Input: part model. Units: mm. Frame: model coordinates. Give positions to 0.01 mm unless a question says otherwise; leave off trailing zeros. Loops run counter-clockwise (first coordinate to the right, second up) from the corner with the lowest first, then second, coordinate; pieces in that order, holes last. Notation, with made-up numbers: (67, 68) -> (111, 68) arc R26 ccw to (111, 94) -> close; hole circle Ø1 at (26.5, 44). An arc over 180 degrees is marked (long way). Answer in a Markdown table with one row per item. Add a question column.
```python
from build123d import *

# Parameters (mm, degrees)
SKETCH1_W           = 17.78
SKETCH1_H           = 33.1
BOSS_EXTRUDE1_DEPTH = 0.8
FILLET1_R           = 0.5
SKETCH2_W           = 9
SKETCH2_H           = 7.3
CUT_EXTRUDE1_DEPTH  = 0.8
SKETCH2_3_W         = 9
SKETCH2_3_H         = 7.3
BOSS_EXTRUDE2_DEPTH = 2.4
SKETCH4_W           = 9
SKETCH4_H           = 2.4
BOSS_EXTRUDE3_DEPTH = 1.524
SKETCH5_W           = 9
SKETCH5_H           = 8.824
BOSS_EXTRUDE4_DEPTH = 0.8
SKETCH6_R           = 0.5
CUT_EXTRUDE2_DEPTH  = 1.524
FILLET2_START       = 8
FILLET2_DEPTH       = 11
FILLET2_START_2     = 16.55
FILLET2_2_DEPTH     = 2.45
CUT_EXTRUDE5_START  = -7.3
CUT_EXTRUDE5_DEPTH  = 7.3


with BuildPart() as part:
    # Sketch1 → Boss-Extrude1 (new body)
    with BuildSketch(Plane(origin=(0, 0, 0), x_dir=(1, 0, 0), z_dir=(0, 1, 0))):
        Rectangle(SKETCH1_W, SKETCH1_H)
    extrude(amount=BOSS_EXTRUDE1_DEPTH)

    # Fillet1
    fillet1_edges = [part.edges().sort_by_distance(p)[0] for p in [
        (-8.89, 0.4, -16.55),
        (8.89, 0.4, -16.55),
        (8.89, 0.4, 16.55),
        (-8.89, 0.4, 16.55),
    ]]
    fillet(fillet1_edges, radius=FILLET1_R)

    # Sketch2 → Cut-Extrude1 (cut)
    with BuildSketch(Plane(origin=(0, 0.8, 0), x_dir=(1, 0, 0), z_dir=(0, 1, 0))):
        with Locations((0, -12.9)):
            Rectangle(SKETCH2_W, SKETCH2_H)
    extrude(amount=-CUT_EXTRUDE1_DEPTH, mode=Mode.SUBTRACT)



with BuildPart() as body_2:
    # Sketch2<3> → Boss-Extrude2 (new body)
    with BuildSketch(Plane(origin=(0, 0.8, 0), x_dir=(1, 0, 0), z_dir=(0, 1, 0))):
        with Locations((0, -12.9)):
            Rectangle(SKETCH2_3_W, SKETCH2_3_H)
    extrude(amount=BOSS_EXTRUDE2_DEPTH)

    # Sketch4 → Boss-Extrude3 (add)
    with BuildSketch(Plane.XY.offset(16.55)):
        with Locations((0, 2)):
            Rectangle(SKETCH4_W, SKETCH4_H)
    extrude(amount=BOSS_EXTRUDE3_DEPTH)


with BuildPart() as part_1:
    add(part.part)

    add(body_2.part)  # Boss-Extrude4 merges body 2
    # Sketch5 → Boss-Extrude4 (add)
    with BuildSketch(Plane.XZ.offset(-0.8)):
        with Locations((0, 13.662)):
            Rectangle(SKETCH5_W, SKETCH5_H)
    extrude(amount=BOSS_EXTRUDE4_DEPTH)

    # Sketch6 → Cut-Extrude2 (cut)
    with BuildSketch(Plane(origin=(0, 0.8, 0), x_dir=(1, 0, 0), z_dir=(0, 1, 0))):
        with Locations(Location((-7.62, 15.28, 0), (0, 0, 270))):
            Circle(SKETCH6_R)
        with Locations(Location((7.62, 15.28, 0), (0, 0, 270))):
            Circle(SKETCH6_R)
        with Locations(Location((7.62, 12.74, 0), (0, 0, 270))):
            Circle(SKETCH6_R)
        with Locations(Location((7.62, 10.2, 0), (0, 0, 270))):
            Circle(SKETCH6_R)
        with Locations(Location((7.62, 7.66, 0), (0, 0, 270))):
            Circle(SKETCH6_R)
        with Locations(Location((7.62, 5.12, 0), (0, 0, 270))):
            Circle(SKETCH6_R)
        with Locations(Location((7.62, 2.58, 0), (0, 0, 270))):
            Circle(SKETCH6_R)
        with Locations(Location((7.62, 0.04, 0), (0, 0, 270))):
            Circle(SKETCH6_R)
        with Locations(Location((7.62, -2.5, 0), (0, 0, 270))):
            Circle(SKETCH6_R)
        with Locations(Location((7.62, -5.04, 0), (0, 0, 270))):
            Circle(SKETCH6_R)
        with Locations(Location((7.62, -7.58, 0), (0, 0, 270))):
            Circle(SKETCH6_R)
        with Locations(Location((7.62, -10.12, 0), (0, 0, 270))):
            Circle(SKETCH6_R)
        with Locations(Location((7.62, -12.66, 0), (0, 0, 270))):
            Circle(SKETCH6_R)
        with Locations(Location((7.62, -15.2, 0), (0, 0, 270))):
            Circle(SKETCH6_R)
        with Locations(Location((-7.62, 12.74, 0), (0, 0, 270))):
            Circle(SKETCH6_R)
        with Locations(Location((-7.62, 10.2, 0), (0, 0, 270))):
            Circle(SKETCH6_R)
        with Locations(Location((-7.62, 7.66, 0), (0, 0, 270))):
            Circle(SKETCH6_R)
        with Locations(Location((-7.62, 5.12, 0), (0, 0, 270))):
            Circle(SKETCH6_R)
        with Locations(Location((-7.62, 2.58, 0), (0, 0, 270))):
            Circle(SKETCH6_R)
        with Locations(Location((-7.62, 0.04, 0), (0, 0, 270))):
            Circle(SKETCH6_R)
        with Locations(Location((-7.62, -2.5, 0), (0, 0, 270))):
            Circle(SKETCH6_R)
        with Locations(Location((-7.62, -5.04, 0), (0, 0, 270))):
            Circle(SKETCH6_R)
        with Locations(Location((-7.62, -7.58, 0), (0, 0, 270))):
            Circle(SKETCH6_R)
        with Locations(Location((-7.62, -10.12, 0), (0, 0, 270))):
            Circle(SKETCH6_R)
        with Locations(Location((-7.62, -12.66, 0), (0, 0, 270))):
            Circle(SKETCH6_R)
        with Locations(Location((-7.62, -15.2, 0), (0, 0, 270))):
            Circle(SKETCH6_R)
    extrude(amount=-CUT_EXTRUDE2_DEPTH, mode=Mode.SUBTRACT)

    # Fillet2: read off the stored shape, not the designer's step
    # Fillet2 outline → Fillet2 (cut)
    with BuildSketch(Plane.XY.offset(FILLET2_START)):
        with BuildLine():
            ThreePointArc((-4.5, 2.2), (-4.207106781, 2.907106781), (-3.5, 3.2))
            Line((-3.5, 3.2), (-4.5, 3.2))
            Line((-4.5, 3.2), (-4.5, 2.2))
        make_face()
        with BuildLine():
            Line((4.5, 3.2), (3.5, 3.2))
            ThreePointArc((3.5, 3.2), (4.207106781, 2.907106781), (4.5, 2.2))
            Line((4.5, 2.2), (4.5, 3.2))
        make_face()
        with BuildLine():
            ThreePointArc((-4.479795897, 0.8), (-4.494936153, 0.899491038), (-4.5, 1))
            Line((-4.5, 1), (-4.5, 0.8))
            Line((-4.5, 0.8), (-4.479795897, 0.8))
        make_face()
        with BuildLine():
            Line((4.5, 0.8), (4.5, 1))
            ThreePointArc((4.5, 1), (4.494936153, 0.899491038), (4.479795897, 0.8))
            Line((4.479795897, 0.8), (4.5, 0.8))
        make_face()
    extrude(amount=FILLET2_DEPTH, mode=Mode.SUBTRACT)

    # Fillet2 2 outline → Fillet2 2 (cut)
    with BuildSketch(Plane.XY.offset(FILLET2_START_2)):
        with BuildLine():
            ThreePointArc((-3.5, 0), (-4.132455532, 0.225403331), (-4.479795897, 0.8))
            Line((-4.479795897, 0.8), (-4.5, 0.8))
            Line((-4.5, 0.8), (-4.5, 0))
            Line((-4.5, 0), (-3.5, 0))
        make_face()
        with BuildLine():
            Line((4.5, 0.8), (4.479795897, 0.8))
            ThreePointArc((4.479795897, 0.8), (4.132455532, 0.225403331), (3.5, 0))
            Line((3.5, 0), (4.5, 0))
            Line((4.5, 0), (4.5, 0.8))
        make_face()
    extrude(amount=FILLET2_2_DEPTH, mode=Mode.SUBTRACT)

    # Sketch7 → Cut-Extrude5 (cut)
    with BuildSketch(Plane.XY.offset(16.55).offset(CUT_EXTRUDE5_START)):
        with BuildLine():
            Line((4.979795897, 0), (4.979795897, 0.8))
            Line((4.979795897, 0.8), (4.479795897, 0.8))
            ThreePointArc((4.479795897, 0.8), (4.132455532, 0.225403331), (3.5, 0))
            Line((3.5, 0), (4.979795897, 0))
        make_face()
        with BuildLine():
            Line((-4.979795897, 0.8), (-4.979795897, 0))
            Line((-4.979795897, 0), (-3.5, 0))
            ThreePointArc((-3.5, 0), (-4.132455532, 0.225403331), (-4.479795897, 0.8))
            Line((-4.479795897, 0.8), (-4.979795897, 0.8))
        make_face()
    extrude(amount=CUT_EXTRUDE5_DEPTH, mode=Mode.SUBTRACT)


solid = part_1.part
```
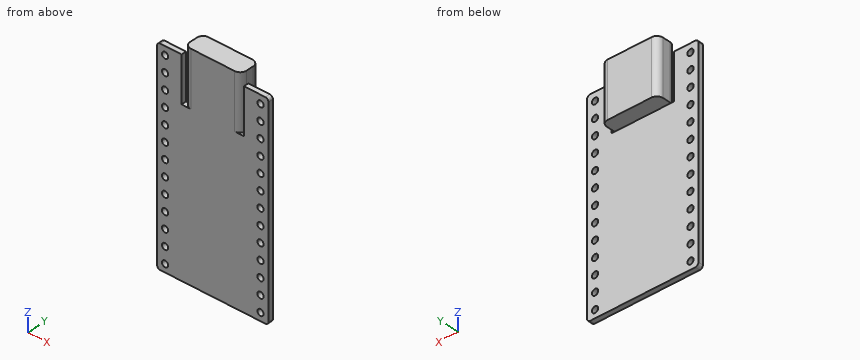
1) Pin query (flat end, axial travel): pin 1 (1 mm diameter, centred on x = 6.5, y = 0.5, fed in from +Z); pin 2 (1 mm diameter, centred on x = -1.5, y = 2, fed in from -Z); pin 3 (1 mm diameter, centred on y = 1.5, z = -0.5, fed in from +X); pin 4 (9 mm diameter, centred on x = 4.5, z = -5, fed in from +Y). Return the tip coordinate at first contact, or that it passes through.
2) Section A-A on z = 10.12. Output: boundary loops of the cut face in (x, y), and give its area (3 significant figures).
3) Section B-B on x = -3. Output: boundary loops of the cut face in (y, z).
4) Section D-D on z = 1. Output: boundary loops of the cut face in (x, y).
5) Material intervals for line 1 along X through (y, z) = (0.7, 7.5); line 2 along X through (y, z) = (0.2, 13); line 3 along Y through (x, z) = (2.5, 2.5), sorted ascending.
6) Section C-C on x = 7.62. State how many separate pieces and enclosed holes the cut face has, and give its area (3 significant figures).
Working result:
| question | item | result |
|---|---|---|
| 1 | pin 1 | stops at z = 16.55 |
| 1 | pin 2 | stops at z = 9.25 |
| 1 | pin 3 | passes through |
| 1 | pin 4 | stops at y = 0.8 |
| 2 | outline | (-8.89, 0) -> (-8.12, 0) -> (-8.12, 0.8) -> (-8.89, 0.8) -> close; (-7.12, 0) -> (-4.98, 0) -> (-4.98, 0.8) -> (-7.12, 0.8) -> close; (-4.5, 1) arc R1 ccw to (-3.5, 0) -> (3.5, 0) arc R1 ccw to (4.5, 1) -> (4.5, 2.2) arc R1 ccw to (3.5, 3.2) -> (-3.5, 3.2) arc R1 ccw to (-4.5, 2.2) -> close; (4.98, 0) -> (7.12, 0) -> (7.12, 0.8) -> (4.98, 0.8) -> close; (8.12, 0) -> (8.89, 0) -> (8.89, 0.8) -> (8.12, 0.8) -> close |
| 2 | area | 32.6 mm2 |
| 3 | outline | (0, -16.55) -> (0.8, -16.55) -> (0.8, 9.25) -> (3.2, 9.25) -> (3.2, 18.07) -> (0, 18.07) -> close |
| 4 | outline | (-8.89, 0) -> (8.89, 0) -> (8.89, 0.8) -> (-8.89, 0.8) -> close |
| 5 | line 1 | x = -8.89 to -8.11, -7.13 to 7.13, 8.11 to 8.89 |
| 5 | line 2 | x = -8.89 to -7.99, -7.25 to -4.98, -4.1 to 4.1, 4.98 to 7.25, 7.99 to 8.89 |
| 5 | line 3 | y = 0 to 0.8 |
| 6 | separate pieces | 14 |
| 6 | enclosed holes | 0 |
| 6 | area | 16.1 mm2 |
